Answer from the drawing. Dimensions are ordinates in mm from the lowest x, y and z of the part. Give positions to 0.01 mm unless a question says otherwise; leave off trailing zeros. Write each loop counter-clockwise with the first axis right and the second up, starting at its lowest first coordinate (ties: lowest second). Pieces come first, ordered by that corner, then holes. Notation, with made-up numbers: (72.25, -29) -> (112.25, -29) arc R13 ccw to (112.25, -22) -> close; hole circle Ø7 at (-30, -9.75). An arc over 180 degrees is marked (long way). Use a Markdown table: item, result. Add a question column.
Q1. Section A-A, the plane z = 2.9 is taken. State how many separate pieces and enclosed holes the cut face has, plus the area to 3 significant figures.
Q2. Section D-D, the plane y = 47 is taken. Give the vertices of the cut face in (x, z).
Q3. Each of these flat-tipped pins is pushed along its axis until it touches: pin 1 Ø10.5 at (x, y) = (271.6, 136) entering from -Z; pin 2 Ø6.5 at (x, y) = (271.6, 160.5) entering from -Z; pin 3 Ø2 at (y, z) = (90.5, 4) entering from +X; pin 4 Ø1.5 at (y, z) = (88.5, 1) entering from +X. Where does it stop, or does it pass through?
Q4. Consider line 1 (Y direction, x = 20, z = 1.5) (1 decimal); line 2 (Y direction, x = 265.5, z = 1.5); line 3 (Y direction, x = 260.5, z = 4) (1 decimal). Determine where each line is inside the solid, lowest interval first.
Q5. Section C-C, the plane x = 238 is taken. Give the vertices of the cut face in (y, z).
Q6. Section B-B, the plane y = 136 is taken. Give the vertices of the cut face in (x, z).
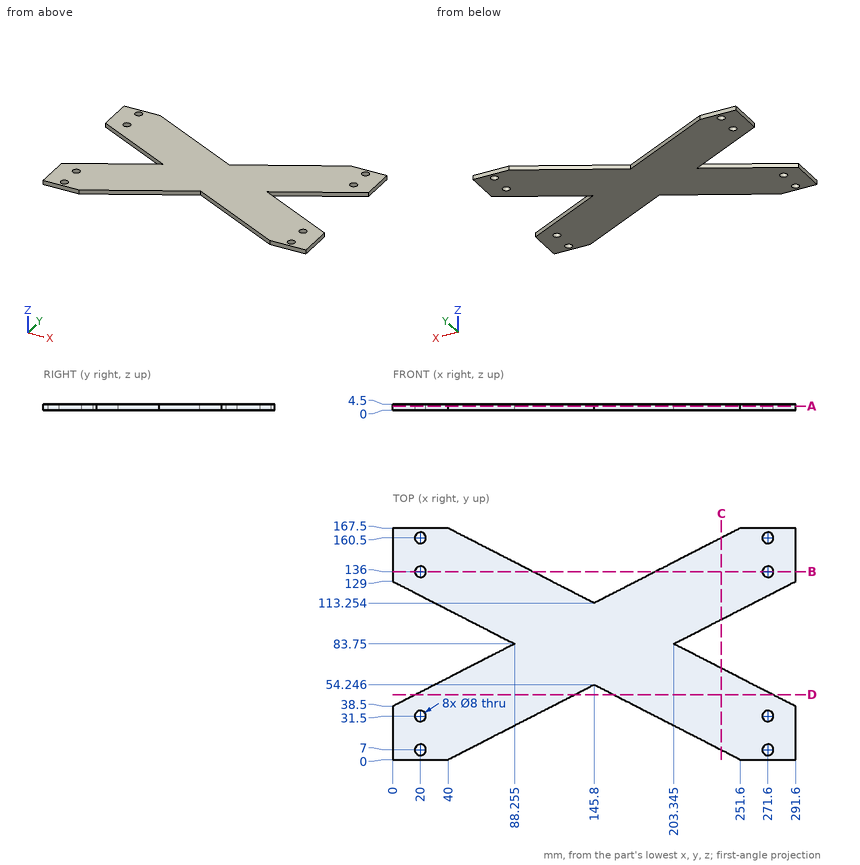
Result set:
| question | item | result |
|---|---|---|
| 1 | separate pieces | 1 |
| 1 | enclosed holes | 8 |
| 1 | area | 29,000 mm2 |
| 2 | outline | (16.58, 0) -> (131.67, 0) -> (131.67, 4.5) -> (16.58, 4.5) -> close; (159.93, 0) -> (275.02, 0) -> (275.02, 4.5) -> (159.93, 4.5) -> close |
| 3 | pin 1 | stops at z = 0 |
| 3 | pin 2 | passes through |
| 3 | pin 3 | stops at x = 218.46 |
| 3 | pin 4 | stops at x = 214.07 |
| 4 | line 1 | y = 0 to 3, 11 to 27.5, 35.5 to 48.8, 118.7 to 132, 140 to 156.5, 164.5 to 167.5 |
| 4 | line 2 | y = 0 to 51.88, 115.62 to 167.5 |
| 4 | line 3 | y = 0 to 54.4, 113.1 to 167.5 |
| 5 | outline | (6.97, 0) -> (65.98, 0) -> (65.98, 4.5) -> (6.97, 4.5) -> close; (101.52, 0) -> (160.53, 0) -> (160.53, 4.5) -> (101.52, 4.5) -> close |
| 6 | outline | (0, 0) -> (16, 0) -> (16, 4.5) -> (0, 4.5) -> close; (24, 0) -> (101.44, 0) -> (101.44, 4.5) -> (24, 4.5) -> close; (190.16, 0) -> (267.6, 0) -> (267.6, 4.5) -> (190.16, 4.5) -> close; (275.6, 0) -> (291.6, 0) -> (291.6, 4.5) -> (275.6, 4.5) -> close |
